For this review, use the dimensioned drawing (mm, ordinates from the lowest corner) and the shaded views. A direction names the side the tool comes from. Coordinates: 2 decimals unless noted, no trailing zeros. Loops run counter-clockwise (first coordinate to the right, second up) from the corner with the lowest first, then second, coordinate; pieces in that order, holes last. Notation, with made-up numbers: (27, -39) - (85, -39) arc R26 cw to (85, -24) - close; hole circle Ø5 at (1.25, 0.5). An arc over 180 degrees is marked (long way). Use one line per item in the form item = value. Start each with the question number.
(1) Add section C-C (y = 4.5). State the section outline as (x, z) points.
(2) Add section B-B (y = 30.75). State the section outline as (x, z) points (1 decimal).
(3) Clearance check with flat-ended pins moving along their axes: pin 1 Ø10 at (y, z) = (12.5, 26.5) entering from -X (1 decimal); pin 2 Ø1 at (x, z) = (21, 4) entering from +Y; pin 3 Ø10 at (x, z) = (22.5, 21) entering from -Y. State where each tip first meets the part, or that it passes through.
(4) Add section D-D (y = 22). State the section outline as (x, z) points, plus the area to 3 significant figures.
(5) For L1, parallel to Y at x = 22, z = 22.1; L2, parallel to X at y = 30, z = 22 (1 decimal); L3, parallel to Z at x = 34, y = 23, list the stretches that pass through material, from the lowest coordinate up.
(6) Tool access review of the marked faces 1, 2 and 3: name each direction out of +Z, -Z, +X, -X, +Y, -Y from which nothing blocks a thin tool from reaching the whole face with its end or side.
(7) Add section A-A (x = 22). State the section outline as (y, z) points.
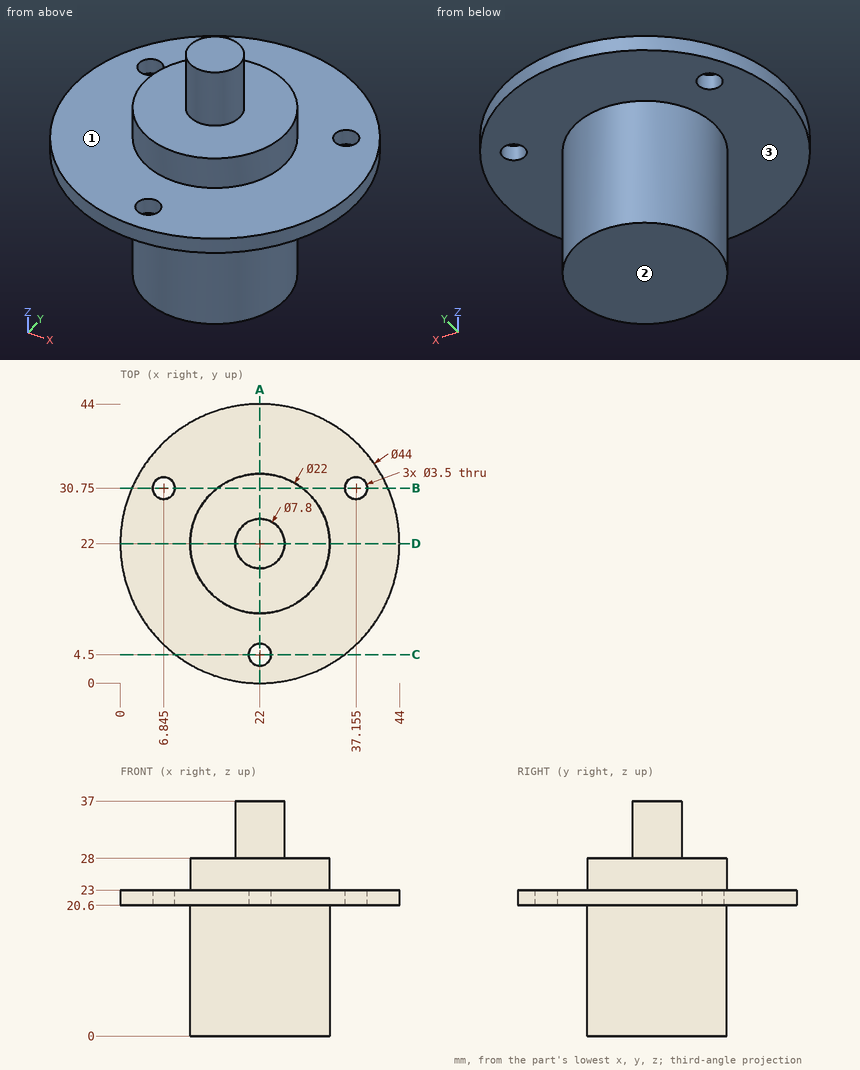
Computed values:
q1.outline = (8.67, 20.6) - (20.25, 20.6) - (20.25, 23) - (8.67, 23) - close; (23.75, 20.6) - (35.33, 20.6) - (35.33, 23) - (23.75, 23) - close
q2.outline = (1.8, 20.6) - (5.1, 20.6) - (5.1, 23) - (1.8, 23) - close; (8.6, 20.6) - (15.3, 20.6) - (15.3, 0) - (28.7, 0) - (28.7, 20.6) - (35.4, 20.6) - (35.4, 23) - (28.7, 23) - (28.7, 28) - (15.3, 28) - (15.3, 23) - (8.6, 23) - close; (38.9, 20.6) - (42.2, 20.6) - (42.2, 23) - (38.9, 23) - close
q3.pin_1 = 0.8
q3.pin_2 = 32.99
q3.pin_3 = 0
q4.outline = (0, 20.6) - (11, 20.6) - (11, 0) - (33, 0) - (33, 20.6) - (44, 20.6) - (44, 23) - (33, 23) - (33, 28) - (25.9, 28) - (25.9, 37) - (18.1, 37) - (18.1, 28) - (11, 28) - (11, 23) - (0, 23) - close
q4.area = 739 mm^2
q5.L1 = 0 to 2.75, 6.25 to 44
q5.L2 = 1.5 to 5.3, 8.4 to 35.6, 38.7 to 42.5
q5.L3 = 20.6 to 23
q6.face_1 = +Z
q6.face_2 = -Z, +X, -X, +Y, -Y
q6.face_3 = -Z
q7.outline = (0, 20.6) - (2.75, 20.6) - (2.75, 23) - (0, 23) - close; (6.25, 20.6) - (11, 20.6) - (11, 0) - (33, 0) - (33, 20.6) - (44, 20.6) - (44, 23) - (33, 23) - (33, 28) - (25.9, 28) - (25.9, 37) - (18.1, 37) - (18.1, 28) - (11, 28) - (11, 23) - (6.25, 23) - close
